Here's how the part is built. I have some questions about the finished solid (model axes, mm). A direction names the side the tool comes from. Coordinates: 2 decimals unless noted, no trailing zeros. Write each loop counter-clockwise with the first axis right and the second up, starting at its lowest first coordinate (ties: lowest second). Pieces come first, ordered by that corner, then holes.
Item 1: If we section it at B-B (y = -17.5): Please give me the cut outline in (x, z) (3 decimals), then the cut area to 3 significant figures.
Item 2: If we section it at D-D (y = 28): Please give me the cut outline in (x, z), then the cut area to 3 significant figures.
Item 3: If I drill on line 1 (X direction, y = -13, z = 2.5); line 2 (X direction, y = 17.5, z = 2.5); line 3 (Y direction, x = 5, z = 4.25), over which ranges is the centre line in solid material (lowest first)?
Item 4: If we section it at A-A (x = 0): Please give me the cut outline in (y, z).
Item 5: For faces 1 (the face through (39.5, -0.1, 3.1)), 2 (the face through (10, 1, 6.35)), which set-ups out of +Z, -Z, +X, -X, +Y, -Y let a thin tool reach every point of the face, with its end or its side?
Item 6: We'd pull the mould along Z, two halves only. Please class faces 3 (the face through (-5.221, 19.186, 3.131)), 4 (the face through (-33.808, -22.369, 3.55)), 5 (the face through (34.01, -22.37, 2.41)), 6 (the face through (10, 1, 0)): +Z half, -Z half, draft (parallel to the pull), parting line (faces both ways), or undercut.
Item 7: I'm going to push flat-ended pins straight in: pin 1 Ø3 at (x, z) = (4.5, 1) entering from -Y; pin 2 Ø1.5 at (x, z) = (13.5, 3.5) entering from +Y; pin 3 Ø3 at (x, z) = (35, 3.175) entering from -Y. Where does each tip first touch, or does it pass through?
Item 8: If we section it at C-C (x = 32): Please give me the cut outline in (y, z), then the cut area to 3 significant figures.
from build123d import *

# Parameters (mm, degrees)
SKETCH_R       = 47.5
PAD_DEPTH      = 6.35
SKETCH001_R    = 4.5
HOLE_DEPTH     = 6.351
SKETCH002_R    = 1.7
HOLE001_DEPTH  = 25
SKETCH003_R    = 1.25
HOLE002_DEPTH  = 25
HOLE002_TIPS_R = 1.25


with BuildPart() as part:
    # Sketch → Pad (new body)
    with BuildSketch(Plane.XY):
        Circle(SKETCH_R)
        with BuildLine():
            ThreePointArc((-38.899906, 6.859103), (-39.5, 0), (-38.899906, -6.859103))
            ThreePointArc((-38.899906, -6.859103), (-33.686855, -10.509321), (-30.036636, -5.296269))
            ThreePointArc((-30.036636, 5.296269), (-30.5, 0), (-30.036636, -5.296269))
            ThreePointArc((-30.036636, 5.296269), (-33.686855, 10.509321), (-38.899906, 6.859103))
        make_face(mode=Mode.SUBTRACT)
        with BuildLine():
            ThreePointArc((30.036636, -5.296269), (30.5, 0), (30.036636, 5.296269))
            ThreePointArc((38.899906, 6.859103), (33.686855, 10.509321), (30.036636, 5.296269))
            ThreePointArc((38.899906, -6.859103), (39.5, 0), (38.899906, 6.859103))
            ThreePointArc((30.036636, -5.296269), (33.686855, -10.509321), (38.899906, -6.859103))
        make_face(mode=Mode.SUBTRACT)
    extrude(amount=PAD_DEPTH)

    # Sketch001 → Hole (cut, through all)
    with BuildSketch(Plane.XY):
        Circle(SKETCH001_R)
    extrude(amount=HOLE_DEPTH, mode=Mode.SUBTRACT)

    # Sketch002 → Hole001 (cut)
    with BuildSketch(Plane.XY):
        with Locations((-5, -17.5)):
            Circle(SKETCH002_R)
        with Locations((5, -17.5)):
            Circle(SKETCH002_R)
        with Locations((5, 17.5)):
            Circle(SKETCH002_R)
        with Locations((-5, 17.5)):
            Circle(SKETCH002_R)
    extrude(amount=HOLE001_DEPTH, mode=Mode.SUBTRACT)

    # Sketch003 → Hole002 (cut)
    with BuildSketch(Plane.XZ.offset(36)):
        with Locations((-35, 3.175)):
            Circle(SKETCH003_R)
        with Locations((35, 3.175)):
            Circle(SKETCH003_R)
    extrude(amount=-HOLE002_DEPTH, mode=Mode.SUBTRACT)

    # Hole002 tips → Hole002 tip 1 section 0
    with BuildSketch(Plane.XZ.offset(11), mode=Mode.PRIVATE) as hole002_tip_1_s0:
        with Locations((-35, 3.175)):
            Circle(HOLE002_TIPS_R)
    loft([hole002_tip_1_s0.sketch, Vertex(-35, -10.248924, 3.175)], mode=Mode.SUBTRACT)

    # Hole002 tips → Hole002 tip 2 section 0
    with BuildSketch(Plane.XZ.offset(11), mode=Mode.PRIVATE) as hole002_tip_2_s0:
        with Locations((35, 3.175)):
            Circle(HOLE002_TIPS_R)
    loft([hole002_tip_2_s0.sketch, Vertex(35, -10.248924, 3.175)], mode=Mode.SUBTRACT)


solid = part.part
Answer list:
1. outline: (-44.159, 0) - (-6.7, 0) - (-6.7, 6.35) - (-44.159, 6.35) - close; (-3.3, 0) - (3.3, 0) - (3.3, 6.35) - (-3.3, 6.35) - close; (6.7, 0) - (44.159, 0) - (44.159, 6.35) - (6.7, 6.35) - close; hole circle Ø2.5 at (-35, 3.175); hole circle Ø2.5 at (35, 3.175)
1. area: 508 mm2
2. outline: (-38.37, 0) - (38.37, 0) - (38.37, 6.35) - (-38.37, 6.35) - close
2. area: 487 mm2
3. line 1: x = -45.69 to -36.05, -33.95 to 33.95, 36.05 to 45.69
3. line 2: x = -44.16 to -6.7, -3.3 to 3.3, 6.7 to 44.16
3. line 3: y = -47.24 to -19.2, -15.8 to 15.8, 19.2 to 47.24
4. outline: (-47.5, 0) - (-4.5, 0) - (-4.5, 6.35) - (-47.5, 6.35) - close; (4.5, 0) - (47.5, 0) - (47.5, 6.35) - (4.5, 6.35) - close
5. face 1: +Z, -Z
5. face 2: +Z, +X, -X, +Y, -Y
6. face 3: draft
6. face 4: undercut
6. face 5: undercut
6. face 6: -Z half
7. pin 1: stops at y = -47.41
7. pin 2: stops at y = 45.76
7. pin 3: stops at y = -33.67
8. outline: (-35.1, 0) - (-9.84, 0) - (-9.84, 6.35) - (-35.1, 6.35) - close; (9.84, 0) - (35.1, 0) - (35.1, 6.35) - (9.84, 6.35) - close
8. area: 321 mm2
